Solid Edge part; units mm, degrees
sketch "Sketch1" plane through (0, 0, 0) normal (0, 0, 1) x (1, 0, 0)
  line L0 (-165.1, -76.2) -> (165.1, -76.2)
  line L1 (165.1, -76.2) -> (165.1, 76.2)
  line L2 (165.1, 76.2) -> (-165.1, 76.2)
  line L3 (-165.1, 76.2) -> (-165.1, -76.2)
  dimension "D1" = 165.1
  dimension "D2" = 165.1
extrude "Protrusion1" add sketch "Sketch1" along normal blind 19.05
sketch "Sketch2" plane through (0, 0, 19.05) normal (0, 0, 1) x (1, 0, 0)
  circle A0 centre (-55.0334, 0) radius 3.9688
extrude "TripodTNutHole" cut sketch "Sketch2" against normal blind 50.8
sketch "Sketch3" plane through (0, 0, 19.05) normal (0, 0, 1) x (1, 0, 0)
  line L0 (99.568, -6.35) -> (150.368, -6.35)
  line L1 (150.368, -6.35) -> (150.368, 6.35)
  line L2 (150.368, 6.35) -> (99.568, 6.35)
  line L3 (99.568, 6.35) -> (99.568, -6.35)
  dimension "D1" = 150.368
  dimension "D2" = 150.368
extrude "ExtrudedCutout_2" cut sketch "Sketch3" against normal blind 25.4
sketch "Sketch4" plane through (0, 0, 19.05) normal (0, 0, 1) x (0, -1, 0)
  circle A0 centre (-32.893, 107.188) radius 3.175
  circle A1 centre (-32.893, 142.748) radius 3.175
  dimension "D1" = 32.893
extrude "MotorMountHoles12" cut sketch "Sketch4" against normal blind 25.4
mirror "Mirror1" about plane through (0, 0, 0) normal (0, -1, 0) of "MotorMountHoles12"
properties material "Wood, Oak"
Could you check a few things on this model? Use its own coordinates, in mm. A direction names the side the tool comes from. Round coordinates to 2 decimals unless told otherwise and drop trailing zeros. Loops run counter-clockwise (first coordinate to the right, second up) from the corner with the lowest first, then second, coordinate; pieces in that order, holes last. Notation, with made-up numbers: M 31,65 L 60,65 A10 cw 60,75 Z; hole C -36.5,-17 d6. An arc over 180 degrees is marked long. Put each result on its own line as item: value.
Q1. Thinking about a two-plate mould opening in X: for faces 3 (the face through (-165.1, 1, 9)), 4 (the face through (-51.248, 1.192, 9.658)), 5 (the face through (2, 76.2, 9)), which applies, released by +X, released by -X, zero draft, split by the parting line, or undercut?
Check result:
face 3: released by -X
face 4: undercut
face 5: zero draft
Q2. Imagine slicing it at C-C (z = 5). Write out the boundary of the cut face in (x, y) (3 decimals), then the cut area to 3 significant figures.
Check result:
outline: M -165.1,-76.2 L 165.1,-76.2 L 165.1,76.2 L -165.1,76.2 Z; hole C -55.033,0 d7.938; hole M 99.568,-6.35 L 150.368,-6.35 L 150.368,6.35 L 99.568,6.35 Z; hole C 107.188,-32.893 d6.35; hole C 107.188,32.893 d6.35; hole C 142.748,-32.893 d6.35; hole C 142.748,32.893 d6.35
area: 49,500 mm2
Q3. Imagine slicing it at A-A (x = 121). Write out the boundary of the cut face in (y, z), then the cut area to 3 significant figures.
Check result:
outline: M -76.2,0 L -6.35,0 L -6.35,19.05 L -76.2,19.05 Z; M 6.35,0 L 76.2,0 L 76.2,19.05 L 6.35,19.05 Z
area: 2,660 mm2
Q4. On a 3-axis mill with a long thin cutter (end or side, diameter ignored), from which of +Z, -Z, +X, -X, +Y, -Y can I reach the whole of each face in a straight line? I mean faces 1 (the face through (99.568, 0, 10)), 2 (the face through (-2, -76.2, 9)). Say none if no direction works.
Check result:
face 1: +Z, -Z
face 2: +Z, -Z, +X, -X, -Y
Q5. For pin 1 (5 mm diameter, centred on x = 142.748, y = -32.893, fed in from +Z); pin 2 (10.5 mm diameter, centred on x = -55.03, y = 0, fed in from -Z), each with a flat end and sliding along its axis, tell me the tip position at first contact or that it passes through.
Check result:
pin 1: through
pin 2: z = 0
Q6. Imagine slicing it at B-B (y = 0). Write out the boundary of the cut face in (x, z), then the cut area to 3 significant figures.
Check result:
outline: M -165.1,0 L -59,0 L -59,19.05 L -165.1,19.05 Z; M -51.06,0 L 99.57,0 L 99.57,19.05 L -51.06,19.05 Z; M 150.37,0 L 165.1,0 L 165.1,19.05 L 150.37,19.05 Z
area: 5,170 mm2
Q7. I need wall thicknesses on probe 1 along X at (y, z) = (6, 2); probe 2 along Y at (x, z) = (118, 9.75); probe 3 along X at (y, z) = (-30.5, 16.5). Which ranges of each line are inside material? Lowest first, please.
Check result:
probe 1: -165.1 to 99.57, 150.37 to 165.1
probe 2: -76.2 to -6.35, 6.35 to 76.2
probe 3: -165.1 to 105.1, 109.27 to 140.66, 144.83 to 165.1
